Could you check a few things on this model? Use its own coordinates, in mm. Face numbers are marked on the shaded views. A direction names the side the tool comes from. Coordinates: 2 decimals unless noted, no trailing zeros. Write each loop counter-clockwise with the first axis right and the second up, starting at its lowest first coordinate (ties: lowest second). Pieces come first, ordered by that corner, then holes. Notation, with made-up numbers: (72.5, 85) - (111.5, 85) arc R9 cw to (111.5, 91) - close; hole circle Ø10 at (24.5, 82). An arc over 180 degrees is marked (long way). Answer as a JSON object with one key per item and string values. Group by question number.
1) Please list where these lines run through material, in increasing order: line 1 along Y through (x, z) = (41, 5.25); line 2 along Y through (x, z) = (50, -0.8); line 3 along X through (y, z) = (-2.75, 4).
2) On a 3-axis mill with a long thin cutter (end or side, diameter ignored), from which of +Z, -Z, +X, -X, +Y, -Y can I reach the whole of each face in a straight line? I mean the marked faces 4 and 5. Say none if no direction works.
3) Will these pins go through, and if not, where does the flat tip stop? pin 1 Ø3 at (x, y) = (50, 0) entering from -Z; pin 2 Ø1 at (x, y) = (24.5, -2.5) entering from +Z; pin 3 Ø1.2 at (y, z) = (6, 4) entering from +X.
4) If we section it at B-B (z = 10.25): Write out the boundary of the cut face in (x, y), plus the area to 3 significant figures.
5) If we section it at C-C (x = 0): Write out the boundary of the cut face in (y, z), plus the area to 3 significant figures.
6) If we section it at A-A (y = 0): State how many separate pieces and enclosed holes the cut face has, plus the area to 3 significant figures.
7) We'd pull the mould along X, two halves only. Please class the marked faces 1, 2 and 3: released by +X, released by -X, zero draft, split by the parting line, or undercut.
8) If we section it at D-D (y = 3.5): Write out the boundary of the cut face in (x, z) (3 decimals), plus the area to 3 significant figures.
```python
from build123d import *

# Parameters (mm, degrees)
SKETCH1_W              = 2
SKETCH1_H              = 2
SKETCH1_H_2            = 10
SKETCH1_W_2            = 59.5
BOSS_EXTRUDE1_DEPTH    = 15
SKETCH1_5_W            = 59.5
SKETCH1_5_H            = 10
SKETCH1_5_R            = 1.75
SKETCH1_5_H_2          = 2
SKETCH1_5_W_2          = 2
BOSS_EXTRUDE2_DEPTH    = 2
SKETCH2_W              = 4
SKETCH2_H              = 2
CUT_EXTRUDE1_DEPTH     = 15
CUT_EXTRUDE2_START     = -14
CUT_EXTRUDE2_OUTLINE_W = 3.7
CUT_EXTRUDE2_OUTLINE_H = 1.5
CUT_EXTRUDE2_DEPTH     = 14
CUT_EXTRUDE3_DEPTH     = 1.5
FILLET1_R              = 2
FILLET2_R              = 1
SKETCH11_W             = 3.7
SKETCH11_H             = 14
BOSS_EXTRUDE4_DEPTH    = 1.5


# Read off the part's stored shape, not the designer's step: Cut-Extrude2
with BuildPart() as part:
    # Sketch1 → Boss-Extrude1 (new body)
    with BuildSketch(Plane.XY):
        with Locations((55.75, 6)):
            Rectangle(SKETCH1_W, SKETCH1_H)
        with Locations((55.75, 0)):
            Rectangle(SKETCH1_W, SKETCH1_H_2)
        with Locations((-5.75, 0)):
            Rectangle(SKETCH1_W, SKETCH1_H_2)
        with Locations((-5.75, 6)):
            Rectangle(SKETCH1_W, SKETCH1_H)
        with Locations((25, 6)):
            Rectangle(SKETCH1_W_2, SKETCH1_H)
        with Locations((-5.75, -6)):
            Rectangle(SKETCH1_W, SKETCH1_H)
        with Locations((25, -6)):
            Rectangle(SKETCH1_W_2, SKETCH1_H)
        with Locations((55.75, -6)):
            Rectangle(SKETCH1_W, SKETCH1_H)
    extrude(amount=BOSS_EXTRUDE1_DEPTH)

    # Sketch1<5> → Boss-Extrude2 (add)
    # profile 1 of 9: a face of its own
    with BuildSketch(Plane.XY):
        with Locations((25, 0)):
            Rectangle(SKETCH1_5_W, SKETCH1_5_H)
        Circle(SKETCH1_5_R, mode=Mode.SUBTRACT)
        with Locations((50, 0)):
            Circle(SKETCH1_5_R, mode=Mode.SUBTRACT)
    # profile 2 of 9: a face of its own
    with BuildSketch(Plane.XY):
        with Locations((25, 6)):
            Rectangle(SKETCH1_5_W, SKETCH1_5_H_2)
    # profile 3 of 9: a face of its own
    with BuildSketch(Plane.XY):
        with Locations((25, -6)):
            Rectangle(SKETCH1_5_W, SKETCH1_5_H_2)
    # profile 4 of 9: a face of its own
    with BuildSketch(Plane.XY):
        with Locations((55.75, 0)):
            Rectangle(SKETCH1_5_W_2, SKETCH1_5_H)
    # profile 5 of 9: a face of its own
    with BuildSketch(Plane.XY):
        with Locations((55.75, 6)):
            Rectangle(SKETCH1_5_W_2, SKETCH1_5_H_2)
    # profile 6 of 9: a face of its own
    with BuildSketch(Plane.XY):
        with Locations((55.75, -6)):
            Rectangle(SKETCH1_5_W_2, SKETCH1_5_H_2)
    # profile 7 of 9: a face of its own
    with BuildSketch(Plane.XY):
        with Locations((-5.75, 6)):
            Rectangle(SKETCH1_5_W_2, SKETCH1_5_H_2)
    # profile 8 of 9: a face of its own
    with BuildSketch(Plane.XY):
        with Locations((-5.75, 0)):
            Rectangle(SKETCH1_5_W_2, SKETCH1_5_H)
    # profile 9 of 9: a face of its own
    with BuildSketch(Plane.XY):
        with Locations((-5.75, -6)):
            Rectangle(SKETCH1_5_W_2, SKETCH1_5_H_2)
    extrude(amount=-BOSS_EXTRUDE2_DEPTH)

    # Sketch2 → Cut-Extrude1 (cut)
    with BuildSketch(Plane.XY.offset(15)):
        with Locations((3.5, -6)):
            Rectangle(SKETCH2_W, SKETCH2_H)
        with Locations((46.5, -6)):
            Rectangle(SKETCH2_W, SKETCH2_H)
    extrude(amount=-CUT_EXTRUDE1_DEPTH, mode=Mode.SUBTRACT)

    # Cut-Extrude2 outline → Cut-Extrude2 (cut)
    with BuildSketch(Plane(origin=(0, 7, 0), x_dir=(1, 0, 0), z_dir=(0, 1, 0)).offset(CUT_EXTRUDE2_START)):
        with Locations((8.35, -4)):
            Rectangle(CUT_EXTRUDE2_OUTLINE_W, CUT_EXTRUDE2_OUTLINE_H)
        with Locations((41.65, -4)):
            Rectangle(CUT_EXTRUDE2_OUTLINE_W, CUT_EXTRUDE2_OUTLINE_H)
    extrude(amount=CUT_EXTRUDE2_DEPTH, mode=Mode.SUBTRACT)

    # Sketch4 → Cut-Extrude3 (cut)
    with BuildSketch(Plane(origin=(0, 0, -2), x_dir=(-1, 0, 0), z_dir=(0, 0, -1))):
        Polygon((-10.125, 7), (-10.125, 5), (-10.125, -5), (-10.125, -7), (-6.425, -7), (-6.425, 7), align=None)
        Polygon((-39.875, 5), (-39.875, 7), (-43.575, 7), (-43.575, -7), (-39.875, -7), (-39.875, -5), align=None)
    extrude(amount=-CUT_EXTRUDE3_DEPTH, mode=Mode.SUBTRACT)

    # Fillet1
    fillet1_edges = [part.edges().sort_by_distance(p)[0] for p in [
        (-6.75, 7, 6.5),
        (56.75, 7, 6.5),
        (56.75, -7, 6.5),
        (-6.75, -7, 6.5),
    ]]
    fillet(fillet1_edges, radius=FILLET1_R)

    # Fillet2
    fillet2_edges = [part.edges().sort_by_distance(p)[0] for p in [
        (10.125, -7, -1.25),
        (10.125, 7, -1.25),
        (6.425, 7, -1.25),
        (6.425, -7, -1.25),
        (39.875, 7, -1.25),
        (39.875, -7, -1.25),
        (43.575, -7, -1.25),
        (43.575, 7, -1.25),
        (1.5, -6, 0),
        (5.5, -6, 0),
        (48.5, -6, 0),
        (44.5, -6, 0),
    ]]
    fillet(fillet2_edges, radius=FILLET2_R)

    # Sketch11 → Boss-Extrude4 (add)
    with BuildSketch(Plane(origin=(0, 0, -0.5), x_dir=(-1, 0, 0), z_dir=(0, 0, -1))):
        with Locations((-41.725, 0)):
            Rectangle(SKETCH11_W, SKETCH11_H)
        with Locations((-8.275, 0)):
            Rectangle(SKETCH11_W, SKETCH11_H)
    extrude(amount=-BOSS_EXTRUDE4_DEPTH)


solid = part.part
```
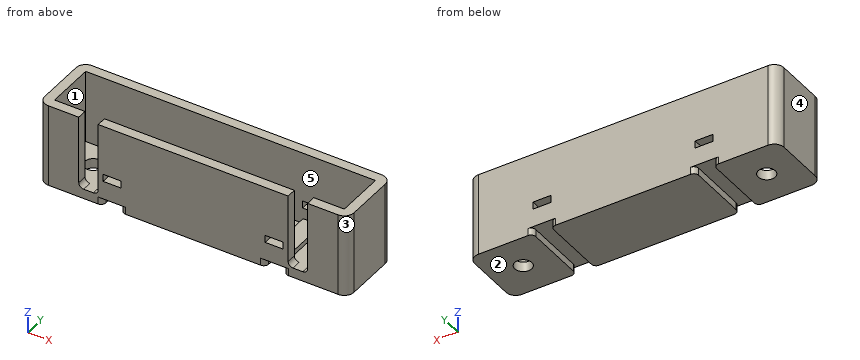
Here are the results:
{
 "1": {"line 1": "y = -7 to -5, 5 to 7", "line 2": "y = -7 to -1.75, 1.75 to 7", "line 3": "x = -6.75 to -4.75, 54.75 to 56.75"},
 "2": {"face 4": "+Z, -Z, -X, +Y, -Y", "face 5": "+Z"},
 "3": {"pin 1": "passes through", "pin 2": "stops at z = 0", "pin 3": "stops at x = 56.71"},
 "4": {"outline": "(-6.75, -5) arc R2 ccw to (-4.75, -7) - (1.5, -7) - (1.5, -5) - (-4.75, -5) - (-4.75, 5) - (54.75, 5) - (54.75, -5) - (48.5, -5) - (48.5, -7) - (54.75, -7) arc R2 ccw to (56.75, -5) - (56.75, 5) arc R2 ccw to (54.75, 7) - (-4.75, 7) arc R2 ccw to (-6.75, 5) - close; (5.5, -7) - (44.5, -7) - (44.5, -5) - (5.5, -5) - close", "area": "275 mm²"},
 "5": {"outline": "(-7, -2) - (-1.75, -2) - (-1.75, 0) - (-5, 0) - (-5, 15) - (-7, 15) - close; (1.75, -2) - (7, -2) - (7, 15) - (5, 15) - (5, 0) - (1.75, 0) - close", "area": "81.0 mm²"},
 "6": {"separate pieces": "3", "enclosed holes": "0", "area": "169 mm²"},
 "7": {"face 1": "undercut", "face 2": "zero draft", "face 3": "released by +X"},
 "8": {"outline": "(-6.75, -2) - (6.425, -2) - (6.425, -0.5) - (10.125, -0.5) - (10.125, -2) - (39.875, -2) - (39.875, -0.5) - (43.575, -0.5) - (43.575, -2) - (56.75, -2) - (56.75, 15) - (54.75, 15) - (54.75, 0) - (43.575, 0) - (43.575, 1) - (39.875, 1) - (39.875, 0) - (10.125, 0) - (10.125, 1) - (6.425, 1) - (6.425, 0) - (-4.75, 0) - (-4.75, 15) - (-6.75, 15) - close", "area": "183 mm²"}
}
